Design review of the part built by this model. Coordinates are the model's own, in mm. A direction names the side the tool comes from. Coordinates: 2 decimals unless noted, no trailing zeros. Loops run counter-clockwise (first coordinate to the right, second up) from the corner with the lowest first, then second, coordinate; pieces in that order, holes last. Notation, with made-up numbers: M 28,57.25 L 62,57.25 A20 cw 62,77.25 Z; hole C 41,-4.5 d1. An arc over 180 degrees is marked long. Answer as a JSON object with one key per item and string values. Group by question number.
1. To check wall thickness, follow probe 1 along X at (y, z) = (2.5, -4.25); probe 2 along Z at (x, y) = (19.5, 2.5); probe 3 along Y at (x, z) = (38, -3). State the ranges of each line that lie inside material, in increasing order.
2. Insertion check: pin 1 (3 mm diameter, centred on x = 31.5, z = -3, fed in from -Y); pin 2 (1.5 mm diameter, centred on x = 18, y = 0, fed in from +Z); pin 3 (3 mm diameter, centred on x = 11, y = 2.5, fed in from -Z). Each pin has a flat end and moves straight along its axis. Give the tip position at first contact, or say it passes through.
3. Consider section A-A (x = 27.5). State the section outline as (y, z) points, then the cut area to 3 significant figures.
4. Machinability: for faces 1 (the flat face through (-0.6, 1, -6)), 2 (the conical face through (-5.2, -6.67, 0.15)), which of the approach directions +Z, -Z, +X, -X, +Y, -Y give a long, thin tool a straight path to every point of the face, cutting with its end or side? Answer none if there is none.
Autodesk Inventor part; units mm, degrees
ref_plane "Work Plane1" through (1.525, 0, 0) normal (0, 0, 1) x (1, 0, 0)
ref_plane "YZ Plane" through (0, 0, 0) normal (1, 0, 0) x (0, 1, 0)
ref_plane "XZ Plane" through (0, 0, 0) normal (0, 1, 0) x (-1, 0, 0)
sketch "Sketch1" plane through (0, 0, 0) normal (0, 0, 1) x (1, 0, 0)
  line L0 (0, 5.815) -> (0, 4)
  line L1 (18, 4) -> (40, 4)
  line L2 (40, 4) -> (40, 0)
  line L3 (40, 0) -> (-0.6001, 0)
  line L4 (-8.7201, 0) -> (48.12, 0)
  line L5 (-0.6001, 0) -> (-0.6001, 5.815)
  line L6 (-0.6001, 5.815) -> (0, 5.815)
  line L7 (18, 4) -> (17.2331, 4)
  line L8 (17.2331, 4) -> (0, 4)
  line L9 (0, -1.163) -> (0, 6.978)
  dimension "d0" = 40
  dimension "d1" = 22
  dimension "d2" = 8
  dimension "d9" = 0.6001
  dimension "d10" = 11.63
  dimension "d13" = 0.7669
  dimension "d14" = 8
revolve "Body" add sketch "Sketch1" angle 360 about axis through (40, 0, 0) along (-1, 0, 0)
sketch "Sketch2" plane through (-0.6001, 0, 0) normal (-1, 0, 0) x (0, 0, 1)
  line L0 (0, 7.5056) -> (6.5, 3.7528)
  line L1 (6.5, 3.7528) -> (6.5, -3.7528)
  line L2 (6.5, -3.7528) -> (0, -7.5056)
  line L3 (0, -7.5056) -> (-6.5, -3.7528)
  line L4 (-6.5, -3.7528) -> (-6.5, 3.7528)
  line L5 (-6.5, 3.7528) -> (0, 7.5056)
  point P0 (0, 0)
  point P1 (0, 0)
  dimension "d11" = 13
extrude "Head" add sketch "Sketch2" along normal blind 4.7
sketch "Sketch4" plane through (0, 0, 0) normal (0, 0, 1) x (1, 0, 0)
  line L0 (-5.3001, 6.5) -> (-5.3001, 7.5056)
  line L1 (-5.3001, 7.5056) -> (-4.7195, 7.5056)
  line L2 (-4.7195, 7.5056) -> (-5.3001, 6.5)
  line L3 (-6.2401, 0) -> (0.3399, 0)
  line L4 (-0.6001, 7.5056) -> (-5.3001, 7.5056)
  line L5 (-5.3001, 3.7528) -> (-5.3001, 7.5056)
  dimension "d5" = 30
  dimension "d19" = 13
revolve "Chamfer1" cut sketch "Sketch4" angle 360 about axis through (-10, 0, 0) along (1, 0, 0)
thread "Thread"
chamfer "Chamfer2" distance 0.7668 distance2 0.7669 1 edges at (40, -4, 0) measured on face at (40, 0.4453, 1.0204)
ref_plane "Work Plane1" through (1.525, 0, 0) normal (0, 0, 1) x (1, 0, 0)
equation "\"d0\" = NLG"
equation "\"d1\" = GEL"
equation "\"d2\" = GD"
equation "\"d10\" = SD2"
equation "\"d14\" = BDM"
equation "\"d11\" = SW"
equation "\"d3\" = KOH - SD"
equation "\"d5\" = ANG1"
equation "\"d19\" = SW0"
equation "\"d15\" = GEL"
equation "\"d6\" = -0.5 * SPD + 0.5 * GD"
equation "\"NLG\" = 40"
equation "\"GD\" = NND"
equation "\"BDM\" = NND"
equation "\"KOH\" = 5.3"
equation "\"GEL\" = 22"
equation "\"SW\" = 13"
equation "\"SW0\" = SW"
equation "\"SPD\" = NND - 1.2269 * PTC"
equation "\"SD2\" = 11.63"
equation "\"SD\" = 0.6"
equation "\"ANG1\" = 30deg"
equation "\"GAL\" = 0.61345 * PTC"
equation "\"GUL\" = 0.61345 * PTC"
equation "\"RR\" = 0.4"
equation "\"GD1\" = THREADDIA - 1.2269 * PTC"
equation "\"THREADDIA\" = 8"
equation "\"SDH\" = SD2"
equation "\"TOA\" = 30deg"
equation "\"PTC\" = 1.25"
equation "\"NND\" = 8"
equation "\"E0\" = 1.155 * SW"
properties part number "ISO 4014 - M8 x 40" material "Stainless Steel, 440C"
Findings below:
{
 "1": {"probe 1": "x = -5.3 to 0", "probe 2": "z = -3.12 to 3.12", "probe 3": "y = -2.65 to 2.65"},
 "2": {"pin 1": "stops at y = -3.71", "pin 2": "stops at z = 4", "pin 3": "stops at z = -3.87"},
 "3": {"outline": "C 0,0 d8", "area": "50.3 mm^2"},
 "4": {"face 1": "+X", "face 2": "-X, -Y"}
}
